Model file for the job. Use its own axes, mm. Face numbers are marked on the shaded views. A direction names the side the tool comes from. Round coordinates to 2 decimals unless told otherwise and drop trailing zeros. Loops run counter-clockwise (first coordinate to the right, second up) from the corner with the lowest first, then second, coordinate; pieces in that order, holes last. Notation, with made-up numbers: (57.25, 67) -> (62.25, 67) arc R14 ccw to (62.25, 93) -> close; hole circle Ø6 at (86.25, 54.25). An arc over 180 degrees is marked (long way). Use a Markdown table: item, result. Add a question column.
Autodesk Inventor part; units mm, degrees
ref_plane "YZ Plane" through (0, 0, 0) normal (1, 0, 0) x (0, 1, 0)
ref_plane "XZ Plane" through (0, 0, 0) normal (0, 1, 0) x (-1, 0, 0)
ref_plane "XY Plane" through (0, 0, 0) normal (0, 0, 1) x (1, 0, 0)
sketch "Esquisse1" plane through (0, 0, 0) normal (0, 1, 0) x (-1, 0, 0)
  line L0 (38, 30) -> (-38, 30)
  line L1 (-38, 30) -> (-38, -30)
  line L2 (-38, -30) -> (38, -30)
  line L3 (38, -30) -> (38, 30)
  line L4 (38, 30) -> (-38, -30) construction
  line L5 (-38, 30) -> (38, -30) construction
  point P0 (0, 0)
  dimension "d0" = 76
  dimension "d1" = 60
extrude "Extrusion1" add sketch "Esquisse1" along normal blind 6
sketch "Esquisse2" plane through (0, 6, 0) normal (0, 1, 0) x (1, 0, 0)
  line L0 (38, 30) -> (-38, 30)
  line L1 (-38, -30) -> (38, -30)
  line L2 (-38, 30) -> (-32, 30)
  line L3 (-32, 30) -> (-32, -30)
  line L4 (-32, -30) -> (-38, -30)
  line L5 (-38, -30) -> (-38, 30)
  line L6 (38, 30) -> (32, 30)
  line L7 (32, 30) -> (32, -30)
  line L8 (32, -30) -> (38, -30)
  line L9 (38, -30) -> (38, 30)
  point P0 (0, 0)
  dimension "d4" = 6
  dimension "d5" = 6
extrude "Extrusion2" add sketch "Esquisse2" along normal blind 14 contours L9 L1 L7 L0 | L3 L1 L5 L0
chamfer "Chanfrein1" distance 2 angle 45 2 edges at (-32, 6, 0) (32, 6, 0)
sketch "Esquisse4" plane through (38, 0, 30) normal (1, 0, 0) x (0, 0, -1)
  line L0 (0, 20) -> (60, 20)
  line L1 (60, 0) -> (60, 20)
  line L2 (0, 0) -> (0, 20)
  line L3 (0, 0) -> (60, 0)
  point P0 (30, 0)
  point P1 (52, 14)
  point P2 (8, 14)
  dimension "d11" = 6
  dimension "d12" = 8
  dimension "d13" = 8
  dimension "d21" = 14
hole "Perçage1" at (38, 14, -22) at (38, 14, 22) direction (-1, 0, 0) diameter 5.5 end through all
properties part number "base_cloison"
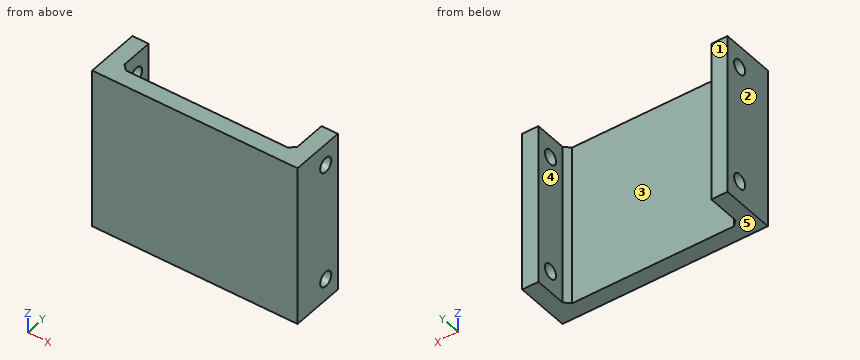
1) Cut at C-C on y = 9.5. Write the cut outline in (x, z), and give its area (3 significant figures).
2) Cut at B-B on z = -22. Write the cut outline in (x, y), and give its area (3 significant figures).
3) Wall check: probe 1 along Z at (x, y) = (-33.5, 14); probe 2 along Y at (x, z) = (-35, 22); probe 3 along X at (y, z) = (17, -26.5). Give the ranges that are in metal, low to high. Write a range as from..to.
4) Cut at D-D on x = 0. Write the cut outline in (y, z).
5) Cut at A-A on y = 14. Write the cut outline in (x, z).
6) Tool access for the marked faces 4 and 5: list every direction of +Z, -Z, +X, -X, +Y, -Y with a clear straight run to the whole face (end or side of a thin tool).
7) Pull direction X, two halves, no side cores. Call the marked faces 1, 2 and 3: +X half, -X half, draft (parallel to the pull), parting line (faces both ways), or undercut.
8) Pin check, flat tip, straight feed: pin 1 Ø5 at (y, z) = (14, -22) entering from +X. Stop position of the tip, or through.
Established:
| question | item | result |
|---|---|---|
| 1 | outline | (-38, -30) -> (-32, -30) -> (-32, 30) -> (-38, 30) -> close; (32, -30) -> (38, -30) -> (38, 30) -> (32, 30) -> close |
| 1 | area | 720 mm^2 |
| 2 | outline | (-38, 0) -> (38, 0) -> (38, 11.25) -> (32, 11.25) -> (32, 8) -> (30, 6) -> (-30, 6) -> (-32, 8) -> (-32, 11.25) -> (-38, 11.25) -> close; (-38, 16.75) -> (-32, 16.75) -> (-32, 20) -> (-38, 20) -> close; (32, 16.75) -> (38, 16.75) -> (38, 20) -> (32, 20) -> close |
| 2 | area | 562 mm^2 |
| 3 | probe 1 | z = -30..-24.75, -19.25..19.25, 24.75..30 |
| 3 | probe 2 | y = 0..11.25, 16.75..20 |
| 3 | probe 3 | x = -38..-32, 32..38 |
| 4 | outline | (0, -30) -> (6, -30) -> (6, 30) -> (0, 30) -> close |
| 5 | outline | (-38, -30) -> (-32, -30) -> (-32, -24.75) -> (-38, -24.75) -> close; (-38, -19.25) -> (-32, -19.25) -> (-32, 19.25) -> (-38, 19.25) -> close; (-38, 24.75) -> (-32, 24.75) -> (-32, 30) -> (-38, 30) -> close; (32, -30) -> (38, -30) -> (38, -24.75) -> (32, -24.75) -> close; (32, -19.25) -> (38, -19.25) -> (38, 19.25) -> (32, 19.25) -> close; (32, 24.75) -> (38, 24.75) -> (38, 30) -> (32, 30) -> close |
| 6 | face 4 | +Z, -Z, +Y |
| 6 | face 5 | -Z, +X, -X, +Y, -Y |
| 7 | face 1 | draft |
| 7 | face 2 | -X half |
| 7 | face 3 | undercut |
| 8 | pin 1 | passes through |
